```python
from build123d import *

# Parameters (mm, degrees)
F1_DEPTH = 75
F3_DEPTH = 100
F5_DEPTH = 100
F6_R     = 13.5
F7_DEPTH = 20


with BuildPart() as f1:
    # F0 (on Top) → F1 (new body)
    with BuildSketch(Plane.XY):
        with BuildLine():
            Line((0, 40), (0, 0))
            Line((0, 0), (15, 0))
            Line((15, 0), (15, 14))
            ThreePointArc((15, 14), (22.5, 21.5), (30, 14))
            Line((30, 14), (30, 0))
            Line((30, 0), (55, 0))
            Line((55, 0), (55, 25))
            Line((55, 25), (75, 25))
            Line((75, 25), (75, 34.031682))
            ThreePointArc((75, 34.031682), (67.175229, 49.898749), (49.823619, 53.350199))
            Line((49.823619, 53.350199), (0, 40))
        make_face()
    extrude(amount=F1_DEPTH)

    # F2 (on face) → F3 (cut, symmetric)
    with BuildSketch(Plane.YZ.offset(55)):
        Polygon((0, 20), (0, 0), (20, 0), align=None)
    extrude(amount=F3_DEPTH, both=True, mode=Mode.SUBTRACT)

    # F4 (on face) → F5 (cut)
    with BuildSketch(Plane.YZ.offset(55)):
        Polygon((0, 42.03419), (20, 45), (0, 55), align=None)
    extrude(amount=-F5_DEPTH, mode=Mode.SUBTRACT)

    # F6 (on face) → F7 (join)
    with BuildSketch(Plane.XY.offset(75)):
        with Locations((59.191159, 39)):
            Circle(F6_R)
    extrude(amount=F7_DEPTH)


solid = f1.part
```
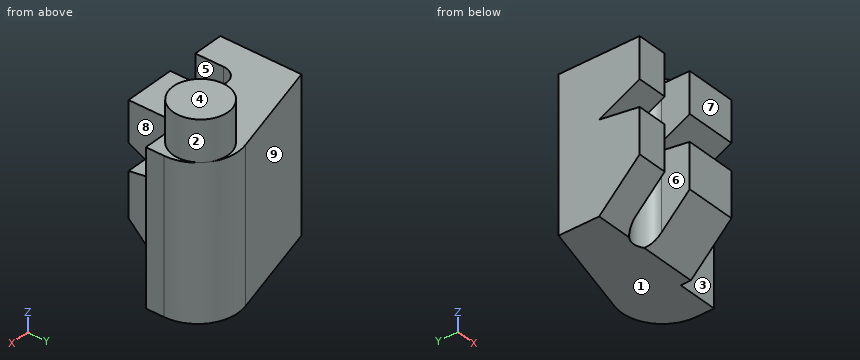
Can you work these out from the model? Positions are in its coordinate system, mm. Face numbers are marked on the shaded views. A direction names the side the tool comes from. Coordinates: 2 decimals unless noted, no trailing zeros. Loops run counter-clockwise (first coordinate to the right, second up) from the corner with the lowest first, then second, coordinate; pieces in that order, holes last. Notation, with made-up numbers: (63, 67.5) -> (102, 67.5) arc R24 cw to (102, 100.5) -> close; hole circle Ø3 at (79, 86.5). An arc over 180 degrees is marked (long way). Put each result on its own line as item: value. Start each with the question number.
Q1. I want a section at A-A (z = 68). Write out the boundary of the cut face in (x, y), plus the area to 3 significant figures.
Q2. I want a section at C-C (x = 52.5). Write out the boundary of the cut face in (y, z).
Q3. Thinking about a two-plate mould opening in X: for the marked faces 6, 7, 8 and 9, which applies, pulls with the +X half, pulls with the -X half, needs draft (parallel to the pull), parting line crosses it, or undercut?
Q4. If I drill on line 1 (X direction, y = 3.5, z = 31.5); line 2 (X direction, y = 20, z = 14); line 3 (Y direction, x = 55.5, z = 41.5), over which ranges is the centre line in solid material (lowest first)? Write a range as [from, to].
Q5. For the marked faces 1, 2, 3, 4 and 5, which set-ups out of +Z, -Z, +X, -X, +Y, -Y let a thin tool reach every point of the face, with its end or its side?
Q6. I'm going to push flat-ended pins straight in: P1, Ø10, axis at x = 64, z = 76, coming from the -Y side; P2, Ø11, axis at y = 9.5, z = 31.5, coming from the +X side; P3, Ø4, axis at x = 37, z = 49.5, coming from the -Y side; P4, Ø10, axis at y = 5.5, z = 80.5, coming from the +X side. Where does each tip first touch, or does it pass through?
Q7. I want a section at D-D (y = 5). Write out the boundary of the cut face in (x, z).
Q8. I want a section at B-B (y = 10.5). Write out the boundary of the cut face in (x, z), plus the area to 3 significant figures.
Taken from the geometry:
1. outline: (0, 0) -> (15, 0) -> (15, 14) arc R7.5 cw to (30, 14) -> (30, 0) -> (55, 0) -> (55, 25) -> (75, 25) -> (75, 34.03) arc R20 ccw to (49.82, 53.35) -> (0, 40) -> close
1. area: 2,800 mm2
2. outline: (0, 20) -> (20, 0) -> (53.87, 0) -> (53.87, 75) -> (50.73, 75) -> (50.73, 95) -> (27.27, 95) -> (27.27, 75) -> (0, 75) -> (0, 55) -> (20, 45) -> (0, 42.03) -> close
3. face 6: undercut
3. face 7: needs draft
3. face 8: pulls with the +X half
3. face 9: pulls with the -X half
4. line 1: x = [0, 15], [30, 55]
4. line 2: x = [0, 18], [27, 55]
4. line 3: y = [25, 54.03]
5. face 1: -Z, +X, -X, +Y, -Y
5. face 2: +Z
5. face 3: +Z, -Z, +X, -Y
5. face 4: +Z, +X, -X, +Y, -Y
5. face 5: +Z, -Z, -Y
6. P1: stops at y = 25
6. P2: stops at x = 55
6. P3: stops at y = 7
6. P4: passes through
7. outline: (0, 15) -> (15, 15) -> (15, 42.78) -> (0, 42.78) -> close; (0, 52.5) -> (15, 52.5) -> (15, 75) -> (0, 75) -> close; (30, 15) -> (55, 15) -> (55, 42.78) -> (30, 42.78) -> close; (30, 52.5) -> (55, 52.5) -> (55, 75) -> (30, 75) -> close
8. outline: (0, 9.5) -> (15, 9.5) -> (15, 43.59) -> (0, 43.59) -> close; (0, 49.75) -> (15, 49.75) -> (15, 75) -> (0, 75) -> close; (30, 9.5) -> (55, 9.5) -> (55, 43.59) -> (30, 43.59) -> close; (30, 49.75) -> (55, 49.75) -> (55, 75) -> (30, 75) -> close
8. area: 2,370 mm2
